Geometry: final body of the model. Coordinates: model frame, mm. A direction names the side the tool comes from. Give positions to 0.01 mm unless a question says otherwise; leave off trailing zeros. Loops run counter-clockwise (first coordinate to the right, second up) from the corner with the lowest first, then second, coordinate; pieces in that order, holes last.
1. Material intervals for line 1 along Y through (x, z) = (0, 3.1); line 2 along X through (y, z) = (9.5, 2.5); line 3 along X through (y, z) = (6, 4.25), sorted ascending.
2. Section B-B, the plane y = 0. Output: boundary loops of the cut face in (x, z).
3. Section D-D, the plane z = 7. Output: boundary loops of the cut face in (x, y).
4. Section A-A, the plane x = 0. State how many separate pieces and enclosed holes the cut face has, then the cut area to 4 significant figures.
5. First-contact query: P1, Ø4, axis at x = 15.5, z = 5.5, coming from the -Y side; P2, Ø5, axis at x = 13, z = 8, coming from the +Y side; P3, Ø9.5, axis at x = 0, y = -17.5, coming from the +Z side. Flat tips, straight axial feed; report the tip coordinate or a pass-through.
6. Section C-C, the plane z = 1.5. Output: boundary loops of the cut face in (x, y).
7. Draft query along X for faces 1 (the face through (-20.633, -15.821, 2.472)), 2 (the face through (12.16, 8.88, 2.47)), 3 (the face through (-12, 6, 5)). Return one class per face: +X half, -X half, draft (parallel to the pull), parting line (faces both ways), or undercut.
8. Access query for faces 4 (the face through (11.923, 3.755, 8.458)), 5 (the face through (-8.2, 2.8, 12)). Directions: +Z, -Z, +X, -X, +Y, -Y. A direction counts if a zero-diameter tool reaches every point of the face in a straight line with its end or side. Return the directions, or none.
from build123d import *

# Parameters (mm, degrees)
F0_R     = 26
F0_R_2   = 3
F0_R_3   = 12.5
F1_DEPTH = 5
F0_R_4   = 8
F2_DEPTH = 12
F3_SIZE  = 0.5


with BuildPart() as f1:
    # F0 (on Top) → F1 (new body)
    with BuildSketch(Plane.XY):
        Circle(F0_R)
        with Locations((0, -17.5)):
            Circle(F0_R_2, mode=Mode.SUBTRACT)
        with Locations((-15.155445, 8.75)):
            Circle(F0_R_2, mode=Mode.SUBTRACT)
        Circle(F0_R_3, mode=Mode.SUBTRACT)
        with Locations((15.155445, 8.75)):
            Circle(F0_R_2, mode=Mode.SUBTRACT)
    extrude(amount=F1_DEPTH)

    # F0 (on Top) → F2 (join)
    with BuildSketch(Plane.XY):
        Circle(F0_R_3)
        Circle(F0_R_4, mode=Mode.SUBTRACT)
    extrude(amount=F2_DEPTH)

    # F3
    f3_edges = [f1.edges().sort_by_distance(p)[0] for p in [
        (-12.5, 0, 12),
        (-8, 0, 12),
        (-26, 0, 5),
        (-3, -17.5, 5),
        (-18.155445, 8.75, 5),
        (-12.5, 0, 5),
        (12.155445, 8.75, 5),
        (-26, 0, 0),
        (-3, -17.5, 0),
        (-18.155445, 8.75, 0),
        (12.155445, 8.75, 0),
        (-8, 0, 0),
    ]]
    chamfer(f3_edges, length=F3_SIZE)


solid = f1.part
Answers below:
1. line 1: y = -26 to -20.5, -14.5 to -8, 8 to 26
1. line 2: x = -24.2 to -18.06, -12.25 to 12.25, 18.06 to 24.2
1. line 3: x = -25.3 to -16.35, -13.96 to -5.29, 5.29 to 13.96, 16.35 to 25.3
2. outline: (-26, 0.5) - (-25.5, 0) - (-8.5, 0) - (-8, 0.5) - (-8, 11.5) - (-8.5, 12) - (-12, 12) - (-12.5, 11.5) - (-12.5, 5.5) - (-13, 5) - (-25.5, 5) - (-26, 4.5) - close; (8, 0.5) - (8.5, 0) - (25.5, 0) - (26, 0.5) - (26, 4.5) - (25.5, 5) - (13, 5) - (12.5, 5.5) - (12.5, 11.5) - (12, 12) - (8.5, 12) - (8, 11.5) - close
3. outline: circle Ø25 at (0, 0); hole circle Ø16 at (0, 0)
4. separate pieces: 3
4. enclosed holes: 0
4. area: 211.5 mm2
5. P1: stops at y = -22.06
5. P2: stops at y = 6.78
5. P3: stops at z = 5.25
6. outline: circle Ø52 at (0, 0); hole circle Ø6 at (-15.16, 8.75); hole circle Ø16 at (0, 0); hole circle Ø6 at (0, -17.5); hole circle Ø6 at (15.16, 8.75)
7. face 1: parting line
7. face 2: undercut
7. face 3: draft
8. face 4: +Z
8. face 5: +Z, +X, -X, +Y, -Y
